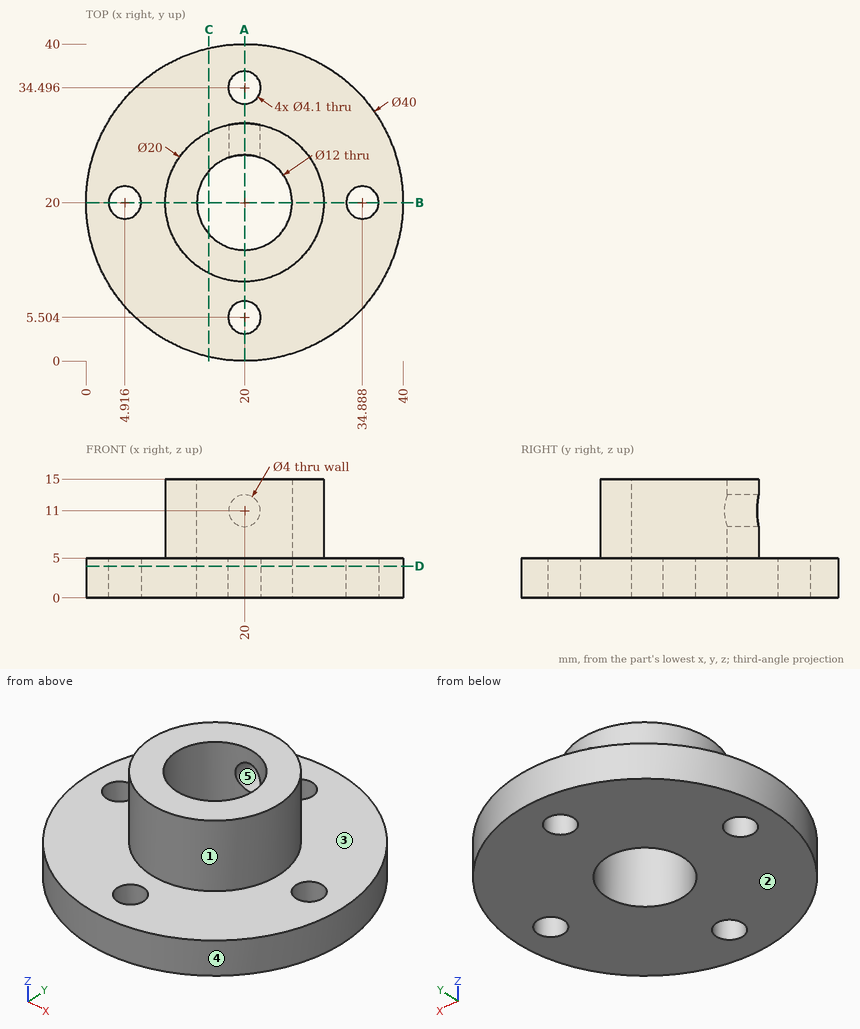
Geometry check sheet. Reference: drawing and pictorial views, mm from the part's lowest x, y, z. A direction names the side the tool comes from. Give positions to 0.01 mm unless a question says otherwise; leave off trailing zeros. Order: outer loops, then holes, each group sorted by start corner. A loop starts at its lowest first (then second) coordinate and runs counter-clockwise, first axis right, second up.
1. Section check A-A, the plane x = 20. Enter the section's corners in (y, z).
2. Access from +Z, -Z, +X, -X, +Y, -Y to the whole of each face (thin tool, end or side, straight path). Record for the marked faces 1 and 2.
3. Release check for a two-part mould opening along X. For the marked faces 3, 4 and 5 record: pulls with the +X half, pulls with the -X half, needs draft (parallel to the pull), parting line crosses it, or undercut.
4. Thickness scan on L1, parallel to Y at x = 20, z = 2.55; L2, parallel to Y at x = 21, z = 4.25 (1 decimal); L3, parallel to Z at x = 10, y = 9. Record the ranges inside material, lowest first.
5. Section check B-B, the plane y = 20. Enter the section's corners in (x, z).
6. Section check D-D, the plane z = 4. Enter the section's corners in (x, y), and give its area (3 significant figures).
7. Section check C-C, the plane x = 15.5. Enter the section's corners in (y, z), and give its area (3 significant figures).
8. Gauge pin test, flat ends, axial feed: pin 1 Ø3.5 at (x, z) = (20, 11) entering from -Y; pin 2 Ø1.5 at (x, z) = (26, 2.5) entering from -Y; pin 3 Ø1 at (x, z) = (18, 12.5) entering from +Y. Record the tip position at first contact, or that the pin passes through.
Values follow:
1. outline: (0, 0) - (3.45, 0) - (3.45, 5) - (0, 5) - close; (7.55, 0) - (14, 0) - (14, 15) - (10, 15) - (10, 5) - (7.55, 5) - close; (26, 0) - (32.45, 0) - (32.45, 5) - (30, 5) - (30, 9) - (26, 9) - close; (26, 13) - (30, 13) - (30, 15) - (26, 15) - close; (36.55, 0) - (40, 0) - (40, 5) - (36.55, 5) - close
2. face 1: +Z
2. face 2: -Z, +X, -X, +Y, -Y
3. face 3: needs draft
3. face 4: parting line crosses it
3. face 5: undercut
4. L1: y = 0 to 3.45, 7.55 to 14, 26 to 32.45, 36.55 to 40
4. L2: y = 0 to 3.7, 7.3 to 14.1, 25.9 to 32.7, 36.3 to 40
4. L3: z = 0 to 5
5. outline: (0, 0) - (2.87, 0) - (2.87, 5) - (0, 5) - close; (6.97, 0) - (14, 0) - (14, 15) - (10, 15) - (10, 5) - (6.97, 5) - close; (26, 0) - (32.84, 0) - (32.84, 5) - (30, 5) - (30, 15) - (26, 15) - close; (36.94, 0) - (40, 0) - (40, 5) - (36.94, 5) - close
6. outline: circle Ø40 at (20, 20); hole circle Ø4.1 at (4.92, 20); hole circle Ø12 at (20, 20); hole circle Ø4.1 at (20, 5.5); hole circle Ø4.1 at (20, 34.5); hole circle Ø4.1 at (34.89, 20)
6. area: 1,090 mm2
7. outline: (0.51, 0) - (16.03, 0) - (16.03, 15) - (11.07, 15) - (11.07, 5) - (0.51, 5) - close; (23.97, 0) - (39.49, 0) - (39.49, 5) - (28.93, 5) - (28.93, 15) - (23.97, 15) - close
7. area: 254 mm2
8. pin 1: stops at y = 10
8. pin 2: stops at y = 0.7
8. pin 3: stops at y = 29.89
